```python
from build123d import *

# Parameters (mm, degrees)
BASE_EXTRUDE_DEPTH = 12.7
LPATTERN1_COUNT    = 2
LPATTERN1_PITCH    = 41.275


with BuildPart() as part:
    # Sketch1 → Base-Extrude (new, symmetric)
    with BuildSketch(Plane.XY):
        with BuildLine():
            Line((-20.6375, 21.1074), (-20.6375, 11.73965134))
            ThreePointArc((-20.6375, 11.73965134), (-19.1389, 9.144), (-20.6375, 6.54834866))
            Line((-20.6375, 6.54834866), (-20.6375, -6.54834866))
            ThreePointArc((-20.6375, -6.54834866), (-19.1389, -9.144), (-20.6375, -11.73965134))
            Line((-20.6375, -11.73965134), (-20.6375, -17.1704))
            ThreePointArc((-20.6375, -17.1704), (-20.198570222, -18.230070222), (-19.1389, -18.669))
            Line((-19.1389, -18.669), (19.1389, -18.669))
            ThreePointArc((19.1389, -18.669), (20.198570222, -18.230070222), (20.6375, -17.1704))
            Line((20.6375, -17.1704), (20.6375, -11.73965134))
            ThreePointArc((20.6375, -11.73965134), (19.1389, -9.144), (20.6375, -6.54834866))
            Line((20.6375, -6.54834866), (20.6375, 6.54834866))
            ThreePointArc((20.6375, 6.54834866), (19.1389, 9.144), (20.6375, 11.73965134))
            Line((20.6375, 11.73965134), (20.6375, 21.1074))
            ThreePointArc((20.6375, 21.1074), (20.198570222, 22.167070222), (19.1389, 22.606))
            Line((19.1389, 22.606), (12.6111, 22.606))
            ThreePointArc((12.6111, 22.606), (11.551429778, 22.167070222), (11.1125, 21.1074))
            Line((11.1125, 21.1074), (11.1125, 16.256))
            Line((11.1125, 16.256), (12.6111, 16.256))
            Line((12.6111, 16.256), (12.6111, 21.1074))
            Line((12.6111, 21.1074), (19.1389, 21.1074))
            Line((19.1389, 21.1074), (19.1389, 12.494971471))
            ThreePointArc((19.1389, 12.494971471), (17.6403, 9.144), (19.1389, 5.793028529))
            Line((19.1389, 5.793028529), (19.1389, -5.793028529))
            ThreePointArc((19.1389, -5.793028529), (17.6403, -9.144), (19.1389, -12.494971471))
            Line((19.1389, -12.494971471), (19.1389, -17.1704))
            Line((19.1389, -17.1704), (-19.1389, -17.1704))
            Line((-19.1389, -17.1704), (-19.1389, -12.494971471))
            ThreePointArc((-19.1389, -12.494971471), (-17.6403, -9.144), (-19.1389, -5.793028529))
            Line((-19.1389, -5.793028529), (-19.1389, 5.793028529))
            ThreePointArc((-19.1389, 5.793028529), (-17.6403, 9.144), (-19.1389, 12.494971471))
            Line((-19.1389, 12.494971471), (-19.1389, 21.1074))
            Line((-19.1389, 21.1074), (-12.6111, 21.1074))
            Line((-12.6111, 21.1074), (-12.6111, 16.256))
            Line((-12.6111, 16.256), (-11.1125, 16.256))
            Line((-11.1125, 16.256), (-11.1125, 21.1074))
            ThreePointArc((-11.1125, 21.1074), (-11.551429778, 22.167070222), (-12.6111, 22.606))
            Line((-12.6111, 22.606), (-19.1389, 22.606))
            ThreePointArc((-19.1389, 22.606), (-20.198570222, 22.167070222), (-20.6375, 21.1074))
        make_face()
    base_extrude = extrude(amount=BASE_EXTRUDE_DEPTH, both=True)

    # LPattern1: Base-Extrude ×2
    with Locations(*[(i * LPATTERN1_PITCH, 0, 0) for i in range(1, LPATTERN1_COUNT)]):
        add(base_extrude)


solid = part.part
```
Model file for the job. Use its own axes, mm. A direction names the side the tool comes from. Coordinates: 2 decimals unless noted, no trailing zeros. Order: outer loops, then holes, each group sorted by start corner. A loop starts at its lowest first (then second) coordinate and runs counter-clockwise, first axis right, second up. Notation, with made-up numbers: (75, 85.25) -> (79, 85.25) arc R10 cw to (79, 102.25) -> close; hole circle Ø5 at (-1, 32.25). An arc over 180 degrees is marked (long way). Answer as a JSON object with one key per item and string values. Group by question number.
1) Cut at B-B, the plane x = 16. Write the cut outline in (y, z), then the cut area to 3 significant figures.
2) Drill centre lines: L1, parallel to X at y = 1, z = -3; L2, parallel to X at y = 11, z = -3.5; L3, parallel to X at y = -9.5, z = -11.5. Where is each one in solid material? Low to high.
3) Cut at D-D, the plane z = 7. Count the separate pieces of the cut face and the enclosed holes in it, then the cut area to 3 significant figures.
4) Flat gauge pins, fed straight in: pin 1 (8 mm diameter, centred on x = 34, y = 13.5, fed in from -Z); pin 2 (4 mm diameter, centred on x = 38.5, z = 2, fed in from +Y). Where does each tip first touch, or does it go through?
5) Cut at C-C, the plane y = 2. Write the cut outline in (x, z).
6) Cut at A-A, the plane y = 18. Write the cut outline in (x, z).
7) Which spindle directions (+Z, -Z, +X, -X, +Y, -Y) get a long thin tool onto all of the face, cutting with end or side? Do faces 1 (the face through (61.485, 22.155, 0.178)), 2 (the face through (19.139, -15, 0)). Say none if no direction does.
8) Pull direction X, two halves, no side cores. Call faces 3 (the face through (-20.638, 16, 0)), 4 (the face through (-19.139, -15, 0)), 5 (the face through (22.136, 0, 0)), 6 (the face through (20, -1, -12.7)): +X half, -X half, draft (parallel to the pull), parting line (faces both ways), or undercut.
Check values:
{
 "1": {"outline": "(-18.67, -12.7) -> (-17.17, -12.7) -> (-17.17, 12.7) -> (-18.67, 12.7) -> close; (21.11, -12.7) -> (22.61, -12.7) -> (22.61, 12.7) -> (21.11, 12.7) -> close", "area": "76.1 mm²"},
 "2": {"L1": "x = -20.64 to -19.14, 19.14 to 22.14, 60.41 to 61.91", "L2": "x = -19.78 to -18.04, 18.04 to 19.78, 21.49 to 23.23, 59.32 to 61.06", "L3": "x = -19.16 to -17.65, 17.65 to 19.16, 22.11 to 23.62, 58.93 to 60.44"},
 "3": {"separate pieces": "1", "enclosed holes": "2", "area": "445 mm²"},
 "4": {"pin 1": "passes through", "pin 2": "stops at y = -17.17"},
 "5": {"outline": "(-20.64, -12.7) -> (-19.14, -12.7) -> (-19.14, 12.7) -> (-20.64, 12.7) -> close; (19.14, -12.7) -> (22.14, -12.7) -> (22.14, 12.7) -> (19.14, 12.7) -> close; (60.41, -12.7) -> (61.91, -12.7) -> (61.91, 12.7) -> (60.41, 12.7) -> close"},
 "6": {"outline": "(-20.64, -12.7) -> (-19.14, -12.7) -> (-19.14, 12.7) -> (-20.64, 12.7) -> close; (-12.61, -12.7) -> (-11.11, -12.7) -> (-11.11, 12.7) -> (-12.61, 12.7) -> close; (11.11, -12.7) -> (12.61, -12.7) -> (12.61, 12.7) -> (11.11, 12.7) -> close; (19.14, -12.7) -> (22.14, -12.7) -> (22.14, 12.7) -> (19.14, 12.7) -> close; (28.66, -12.7) -> (30.16, -12.7) -> (30.16, 12.7) -> (28.66, 12.7) -> close; (52.39, -12.7) -> (53.89, -12.7) -> (53.89, 12.7) -> (52.39, 12.7) -> close; (60.41, -12.7) -> (61.91, -12.7) -> (61.91, 12.7) -> (60.41, 12.7) -> close"},
 "7": {"face 1": "+Z, -Z, +X, +Y", "face 2": "+Z, -Z"},
 "8": {"face 3": "-X half", "face 4": "undercut", "face 5": "undercut", "face 6": "draft"}
}
